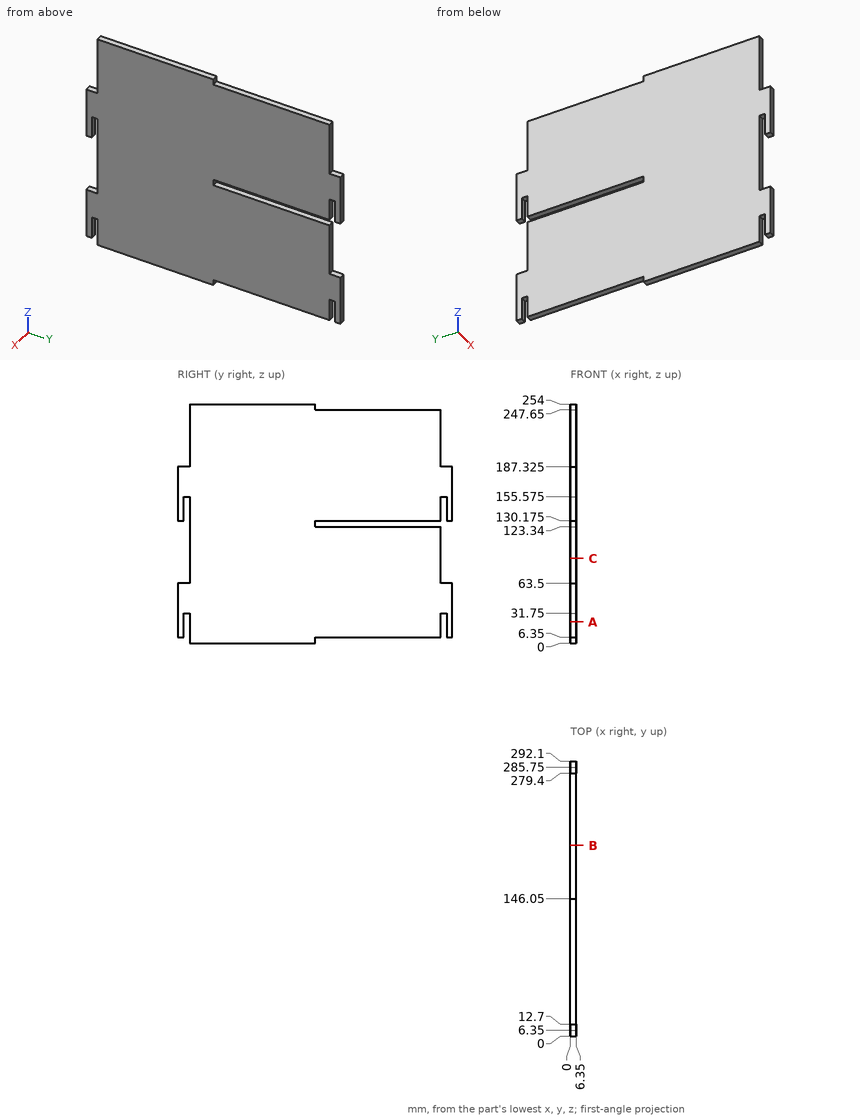
Answer from the drawing. Dimensions are ordinates in mm from the lowest x, y and z of the part. Give positions to 0.01 mm unless a question says otherwise; leave off trailing zeros. Write each loop counter-clockwise with the first axis right and the second up, starting at its lowest first coordinate (ties: lowest second). Pieces come first, ordered by that corner, then holes. Notation, with made-up numbers: (31.25, 44.25) - (76.25, 44.25) arc R11 cw to (76.25, 64.25) - close; hole circle Ø7 at (-23, 9.25). An arc over 180 degrees is marked (long way). Answer in a Markdown table with one row per item. Add a question column.
Item 1: Flat-ended cylindrical pins translate along their axes: P1, Ø3, axis at x = 5.5, z = 189.5, coming from the -Y side; P2, Ø1.9, axis at x = 4, z = 128.5, coming from the +Y side; P3, Ø3, axis at x = 4, y = 5, coming from the -Z side. Find the tip coordinate at first contact, or state that the pin passes through.
Item 2: Section B-B, the plane y = 202.5 is taken. Write down the section's boundary in (x, z) (3 decimals).
Item 3: Section A-A, the plane z = 22.5 is taken. Write down the section's boundary in (x, y), and give its area (3 significant figures).
Item 4: Find the intervals of material crossed by L1, parallel to Y at x = 3.5, z = 24.5; L2, parallel to Z at x = 3, y = 151 (3 decimals); L3, parallel to Y at x = 3.75, z = 203.5, in increasing order.
Item 5: Section C-C, the plane z = 90 is taken. Write down the section's boundary in (x, y).
Recorded:
| question | item | result |
|---|---|---|
| 1 | P1 | stops at y = 12.7 |
| 1 | P2 | stops at y = 146.05 |
| 1 | P3 | stops at z = 6.35 |
| 2 | outline | (0, 6.35) - (6.35, 6.35) - (6.35, 123.34) - (0, 123.34) - close; (0, 130.175) - (6.35, 130.175) - (6.35, 247.65) - (0, 247.65) - close |
| 3 | outline | (0, 0) - (6.35, 0) - (6.35, 6.35) - (0, 6.35) - close; (0, 12.7) - (6.35, 12.7) - (6.35, 279.4) - (0, 279.4) - close; (0, 285.75) - (6.35, 285.75) - (6.35, 292.1) - (0, 292.1) - close |
| 3 | area | 1,770 mm2 |
| 4 | L1 | y = 0 to 6.35, 12.7 to 279.4, 285.75 to 292.1 |
| 4 | L2 | z = 6.35 to 123.34, 130.175 to 247.65 |
| 4 | L3 | y = 12.7 to 279.4 |
| 5 | outline | (0, 12.7) - (6.35, 12.7) - (6.35, 279.4) - (0, 279.4) - close |
